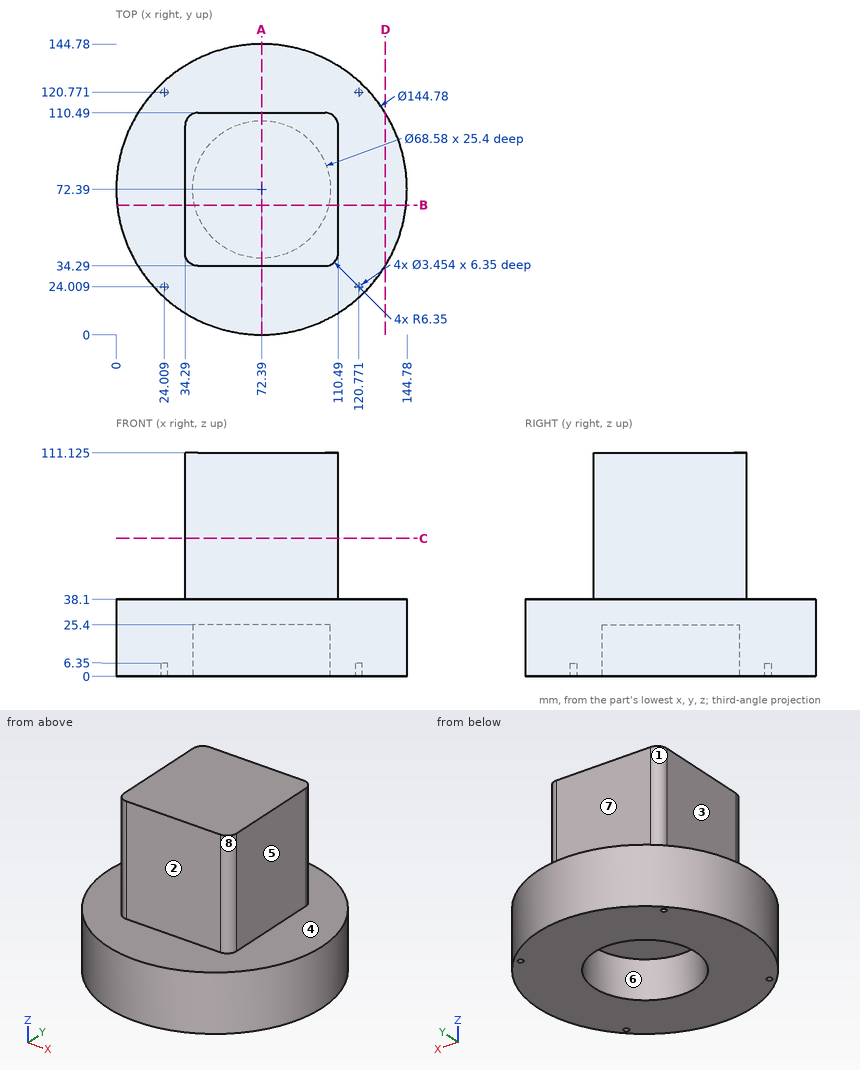
Design review of the part shown in the three views and the two pictorial views. Dimensions are in mm from the part's minimum x, y and z. A direction names the side the tool comes from. Round coordinates to 2 decimals unless told otherwise and drop trailing zeros. Loops run counter-clockwise (first coordinate to the right, second up) from the corner with the lowest first, then second, coordinate; pieces in that order, holes last. Notation, with made-up numbers: (-36.5, 87) - (9.5, 87) arc R20 ccw to (9.5, 97) - close; hole circle Ø1 at (29.25, 48). An arc over 180 degrees is marked (long way). Use CSV: the item, a comma, the result in double quotes.
(1) Machinability: for the marked faces 1, 2, 3, 4 and 5, which of the approach directions +Z, -Z, +X, -X, +Y, -Y give a long, thin tool a straight path to every point of the face, cutting with its end or side? Answer none if there is none.
Working result:
face 1,"+Z, -X, +Y"
face 2,"+Z, +X, -X, -Y"
face 3,"+Z, -X, +Y, -Y"
face 4,"+Z"
face 5,"+Z, +X, +Y, -Y"
(2) Clearance check with flat-ended pins moving along their axes: P1, Ø1.5, axis at y = 125, z = 36, coming from the +X side (1 decimal); P2, Ø4, axis at x = 24.5, y = 16.5, coming from the +Z side; P3, Ø19, axis at x = 74, z = 68, coming from the +Y side. State where each tip first meets the part, or that it passes through.
Working result:
P1,"stops at x = 122.9"
P2,"stops at z = 38.1"
P3,"stops at y = 110.49"
(3) For line 1 (Z direction, x = 24, y = 20); line 2 (Y direction, x = 68.5, z = 55); line 3 (Y direction, x = 87, z = 8), list the stretches that pass through material, from the lowest coordinate up.
Working result:
line 1,"z = 0 to 38.1"
line 2,"y = 34.29 to 110.49"
line 3,"y = 1.49 to 41.37, 103.41 to 143.29"
(4) Take a section at A-A, the plane x = 72.39. Give the boundary of the cut face in (y, z) (1 decimal), plus the area to 3 significant figures.
Working result:
outline,"(0, 0) - (38.1, 0) - (38.1, 25.4) - (106.7, 25.4) - (106.7, 0) - (144.8, 0) - (144.8, 38.1) - (110.5, 38.1) - (110.5, 111.1) - (34.3, 111.1) - (34.3, 38.1) - (0, 38.1) - close"
area,"9,340 mm^2"
(5) Take a section at C-C, the plane z = 68.5. Give the boundary of the cut face in (x, y).
Working result:
outline,"(34.29, 40.64) arc R6.35 ccw to (40.64, 34.29) - (104.14, 34.29) arc R6.35 ccw to (110.49, 40.64) - (110.49, 104.14) arc R6.35 ccw to (104.14, 110.49) - (40.64, 110.49) arc R6.35 ccw to (34.29, 104.14) - close"
(6) The part is to be moulded in two halves that separate along X. For the marked faces 6, 7 and 8, say which applies: pulls with the +X half, pulls with the -X half, needs draft (parallel to the pull), parting line crosses it, or undercut.
Working result:
face 6,"undercut"
face 7,"needs draft"
face 8,"pulls with the +X half"
(7) Take a section at B-B, the plane y = 64.5. Give the boundary of the cut face in (x, z) (1 decimal), plus the area to 3 significant figures.
Working result:
outline,"(0.4, 0) - (39, 0) - (39, 25.4) - (105.8, 25.4) - (105.8, 0) - (144.3, 0) - (144.3, 38.1) - (110.5, 38.1) - (110.5, 111.1) - (34.3, 111.1) - (34.3, 38.1) - (0.4, 38.1) - close"
area,"9,350 mm^2"
(8) Take a section at D-D, the plane x = 134. Give the boundary of the cut face in (y, z).
Working result:
outline,"(34.38, 0) - (110.4, 0) - (110.4, 38.1) - (34.38, 38.1) - close"
